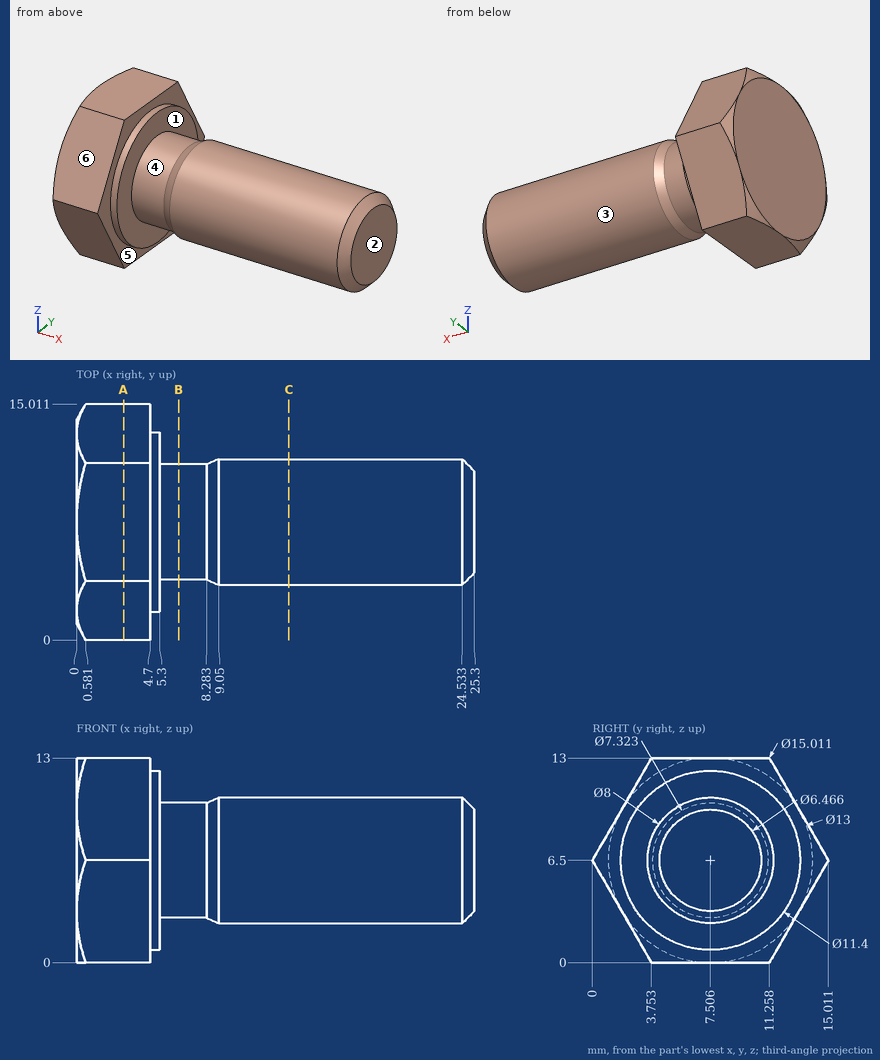
Job drawing, mm, ordinate dimensions from the low corner. One solid piece. A direction names the side the tool comes from. Coordinates: 2 decimals unless noted, no trailing zeros. Order: outer loops, then holes, each group sorted by start corner. A loop starts at its lowest first (then second) coordinate and runs counter-clockwise, first axis right, second up. Notation, with made-up numbers: (-7, 26.25) - (47, 26.25) arc R31 ccw to (47, 62.25) - close; hole circle Ø1 at (-8, 16.5). An arc over 180 degrees is marked (long way). Use CSV: the item, a comma, the result in double quotes.
Item 1: Saw through at C-C on x = 13.5. Give the cut face in (y, z) (1 decimal).
Solved:
outline,"circle Ø8 at (7.5, 6.5)"
Item 2: 3-axis set-ups, long thin cutter, end or side, ignore diameter. For the marked faces 1, 2 and 3: which of +Z, -Z, +X, -X, +Y, -Y reach the whole face in a straight line?
Solved:
face 1,"none"
face 2,"+Z, -Z, +X, +Y, -Y"
face 3,"+X"
Item 3: Drop flat-ended pins along their axis: P1, Ø8, axis at x = 17.5, y = 8, coming from the -Z side; P2, Ø1, axis at x = 4, y = 12, coming from the +Z side; P3, Ø3, axis at x = 22.5, z = 2.5, coming from the -Y side; P4, Ø4, axis at y = 10, z = 3.5, coming from the +X side. Give the stop position or say it passes through.
Solved:
P1,"stops at z = 2.5"
P2,"stops at z = 12.58"
P3,"stops at y = 4.38"
P4,"stops at x = 25.3"
Item 4: Mould opens along X. For the marked faces 4, 5 and 6 say: +X half, -X half, draft (parallel to the pull), parting line (faces both ways), or undercut.
Solved:
face 4,"undercut"
face 5,"+X half"
face 6,"draft"
Item 5: Saw through at A-A on x = 3. Give the cut face in (y, z), and give its area (3 significant figures).
Solved:
outline,"(0, 6.5) - (3.75, 0) - (11.26, 0) - (15.01, 6.5) - (11.26, 13) - (3.75, 13) - close"
area,"146 mm²"
Item 6: Saw through at B-B on x = 6.5. Give the cut face in (y, z) (1 decimal).
Solved:
outline,"circle Ø7.3 at (7.5, 6.5)"
Item 7: Probe probe 1 along X at (y, z) = (7.75, 1.75); probe 2 along X at (y, z) = (5.75, 0.5); probe 3 along X at (y, z) = (11, 5.25) (1 decimal). List the from-to ranges inside material, lowest first.
Solved:
probe 1,"x = 0 to 5.3"
probe 2,"x = 0 to 4.7"
probe 3,"x = 0 to 5.3, 8.4 to 24.8"
